Autodesk Inventor part; units mm, degrees
ref_plane "YZ Plane" through (0, 0, 0) normal (1, 0, 0) x (0, 1, 0)
ref_plane "XZ Plane" through (0, 0, 0) normal (0, 1, 0) x (-1, 0, 0)
ref_plane "XY Plane" through (0, 0, 0) normal (0, 0, 1) x (1, 0, 0)
sketch "Sketch1" plane through (0, 0, 0) normal (0, 1, 0) x (-1, 0, 0)
  line L0 (0, 0) -> (0, -85.725)
  line L1 (15.875, -101.6) -> (101.6, -101.6)
  line L2 (101.6, -101.6) -> (101.6, -88.9)
  line L3 (101.6, -88.9) -> (12.7, -88.9)
  line L4 (12.7, -88.9) -> (12.7, 0)
  line L5 (12.7, 0) -> (0, 0)
  arc A0 (0, -85.725) -> (15.875, -101.6) centre (15.875, -85.725) ccw
  arc A1 (0, -85.725) -> (15.875, -101.6) centre (15.875, -85.725) ccw
  point P0 (0, -101.6)
  dimension "d0" = 101.6
  dimension "d1" = 101.6
  dimension "d2" = 12.7
  dimension "d3" = 12.7
  dimension "d4" = 15.875
  dimension "d5" = 15.875
extrude "Extrusion1" add sketch "Sketch1" along normal blind 101.6
sketch "Sketch2" plane through (-12.7, 0, -88.9) normal (-1, 0, 0) x (0, 0, 1)
  circle A0 centre (50.8, 25.4) radius 6.35
  circle A1 centre (50.8, 76.2) radius 6.35
  line L0 (0, 0) -> (88.9, 0)
  line L1 (88.9, 0) -> (88.9, 101.6)
  dimension "d8" = 12.7
  dimension "d9" = 12.7
  dimension "d10" = 25.4
  dimension "d11" = 50.8
  dimension "d12" = 38.1
  dimension "d13" = 38.1
extrude "Extrusion2" cut sketch "Sketch2" against normal blind 101.6
sketch "Sketch3" plane through (-101.6, 0, -88.9) normal (0, 0, 1) x (1, 0, 0)
  circle A0 centre (38.1, 50.8) radius 12.7
  line L0 (0, 0) -> (0, 101.6)
  line L1 (0, 101.6) -> (88.9, 101.6)
  point P0 (101.6, 0)
  dimension "d16" = 25.4
  dimension "d17" = 38.1
  dimension "d18" = 50.8
extrude "Extrusion3" cut sketch "Sketch3" against normal blind 101.6
fillet "Fillet1" radius 3.175 1 edges at (-12.7, 50.8, -88.9)
properties part number "Soporte"
Could you check a few things on this model? Use its own coordinates, in mm. A direction names the side the tool comes from. Round coordinates to 2 decimals unless told otherwise and drop trailing zeros. Order: outer loops, then holes, each group sorted by start corner. A loop starts at its lowest first (then second) coordinate and runs counter-clockwise, first axis right, second up.
(1) Please list where these lines run through material, in increasing order: line 1 along Y through (x, z) = (-63.5, -97.5); line 2 along Y through (x, z) = (-5.75, -38.1); line 3 along X through (y, z) = (23, -69).
Response values:
line 1: y = 0 to 38.1, 63.5 to 101.6
line 2: y = 0 to 19.05, 31.75 to 69.85, 82.55 to 101.6
line 3: x = -12.7 to 0
(2) Which directions (+Z, -Z, +X, -X, +Y, -Y) give clear straight access to the entire face, cutting with the end or side of a thin tool? Please do faces 5 (the flat face through (-12.7, 50, -43)), 6 (the flat face through (-6, 50, 0)).
Response values:
face 5: +Z, -X, +Y, -Y
face 6: +Z, +X, -X, +Y, -Y
(3) Imagine slicing it at A-A (x = -63.5). Write out the boundary of the cut face in (y, z).
Response values:
outline: (0, -101.6) - (38.1, -101.6) - (38.1, -88.9) - (0, -88.9) - close; (63.5, -101.6) - (101.6, -101.6) - (101.6, -88.9) - (63.5, -88.9) - close
(4) Imagine slicing it at C-C (y = 50.8). Write out the boundary of the cut face in (x, z) (3 decimals).
Response values:
outline: (-101.6, -101.6) - (-76.2, -101.6) - (-76.2, -88.9) - (-101.6, -88.9) - close; (-50.8, -101.6) - (-15.875, -101.6) arc R15.875 ccw to (0, -85.725) - (0, 0) - (-12.7, 0) - (-12.7, -85.725) arc R3.175 cw to (-15.875, -88.9) - (-50.8, -88.9) - close
(5) If we mould it in two halves opening along Y, with no side actions, what happens to faces 1 (the cylindrical face through (-51.768, 45.936, -95.161)), 2 (the flat face through (-9, 101.6, -73)), 3 (the cylindrical face through (-4.8, 50.1, -97.1)), 4 (the cylindrical face through (-6.439, 22.968, -32.234))? For each: released by +Y, released by -Y, zero draft, split by the parting line, or undercut.
Response values:
face 1: undercut
face 2: released by +Y
face 3: zero draft
face 4: undercut
(6) Imagine slicing it at D-D (y = 9). Write out the boundary of the cut face in (x, z) (3 decimals).
Response values:
outline: (-101.6, -101.6) - (-15.875, -101.6) arc R15.875 ccw to (0, -85.725) - (0, 0) - (-12.7, 0) - (-12.7, -85.725) arc R3.175 cw to (-15.875, -88.9) - (-101.6, -88.9) - close
(7) Imagine slicing it at B-B (z = -38.1). Write out the boundary of the cut face in (x, y).
Response values:
outline: (-12.7, 0) - (0, 0) - (0, 19.05) - (-12.7, 19.05) - close; (-12.7, 31.75) - (0, 31.75) - (0, 69.85) - (-12.7, 69.85) - close; (-12.7, 82.55) - (0, 82.55) - (0, 101.6) - (-12.7, 101.6) - close
(8) I'm going to push flat-ended pins straight in: pin 1 (12 mm diameter, centred on x = -22, y = 69, fed in from +Z); pin 2 (20.5 mm diameter, centred on y = 25.4, z = -38.1, fed in from -X). Where does each tip first touch, or does it pass through?
Response values:
pin 1: stops at z = -88.9
pin 2: stops at x = -12.7
